Input: part model. Units: mm. Frame: model coordinates. A direction names the side the tool comes from. Round coordinates to 2 decimals unless told otherwise and drop trailing zeros. Loops run counter-clockwise (first coordinate to the right, second up) from the corner with the lowest first, then second, coordinate; pieces in that order, holes last. Notation, with made-up numbers: (43.5, 84.25) -> (56.5, 84.25) arc R27 cw to (56.5, 100.25) -> close; hole circle Ø5 at (6.25, 15.5). An arc over 180 degrees is marked (long way). Answer as a JSON object with one key per item and string values.
```python
from build123d import *

# Parameters (mm, degrees)
SKETCH_1_R               = 100
SKETCH_1_R_2             = 80
EXTRUDE_1_DEPTH          = 10
SKETCH_3_R               = 1.6
CUT_EXTRUDE_2_DEPTH      = 142.774468788
CUT_EXTRUDE_3_DEPTH      = 3
PATTERN_CIRCULAR_1_COUNT = 3


with BuildPart() as part:
    # 草图1 → 凸台-拉伸1 (new body)
    with BuildSketch(Plane(origin=(0, 0, 0), x_dir=(1, 0, 0), z_dir=(0, 1, 0))):
        with Locations(Location((0, 0, 0), (0, 0, 270))):
            Circle(SKETCH_1_R)
        with Locations(Location((0, 0, 0), (0, 0, 270))):
            Circle(SKETCH_1_R_2, mode=Mode.SUBTRACT)
    extrude(amount=EXTRUDE_1_DEPTH)

    # 草图3 → 切除-拉伸2 (cut, through all)
    with BuildSketch(Plane(origin=(0, 10, 0), x_dir=(1, 0, 0), z_dir=(0, 1, 0))):
        with Locations(Location((-62.39260708, 68.252564653, 0), (0, 0, 270))):
            Circle(SKETCH_3_R)
        with Locations(Location((-84.573353466, 37.397832605, 0), (0, 0, 270))):
            Circle(SKETCH_3_R)
    cut_extrude_2 = extrude(amount=-CUT_EXTRUDE_2_DEPTH, mode=Mode.SUBTRACT)

    # 草图4 → 切除-拉伸3 (cut)
    with BuildSketch(Plane.XZ):
        Polygon((-80.877120495, -38.81834724), (-83.152838831, -33.701599634), (-88.269586436, -35.97731797), (-85.993868101, -41.094065575), align=None)
        Polygon((-62.126188983, -72.20339006), (-66.343432487, -68.51898275), (-62.659025177, -64.301739246), (-58.441781673, -67.986146556), align=None)
    cut_extrude_3 = extrude(amount=-CUT_EXTRUDE_3_DEPTH, mode=Mode.SUBTRACT)

    # 阵列(圆周)1: 切除-拉伸2, 切除-拉伸3 ×3 about axis
    pattern_circular_1_axis = Axis((0, 0, 0), (0, 1, 0))
    add([cut_extrude_2.rotate(pattern_circular_1_axis, i * 360 / PATTERN_CIRCULAR_1_COUNT) for i in range(1, PATTERN_CIRCULAR_1_COUNT)], mode=Mode.SUBTRACT)
    add([cut_extrude_3.rotate(pattern_circular_1_axis, i * 360 / PATTERN_CIRCULAR_1_COUNT) for i in range(1, PATTERN_CIRCULAR_1_COUNT)], mode=Mode.SUBTRACT)


solid = part.part
```
1) Contact query for flat-ended pins moving along their axis: P1, Ø2, axis at x = -28, z = 90, coming from the -Y side; P2, Ø4, axis at y = 7.5, z = 38.5, coming from the -X side; P3, Ø2, axis at x = -57.5, z = 76, coming from the -Y side; P4, Ø4, axis at x = 54, y = 4.5, coming from the -Z side. Output: stop coordinate, or through.
Output:
{"P1": "stops at y = 3", "P2": "stops at x = -93.1", "P3": "stops at y = 0", "P4": "stops at z = -85.42"}
2) Section B-B, the plane x = 0. Output: boundary loops of the cut face in (y, z), plus the area to 3 significant figures.
Output:
{"outline": "(0, -100) -> (10, -100) -> (10, -80) -> (0, -80) -> close; (0, 80) -> (10, 80) -> (10, 100) -> (0, 100) -> close", "area": "400 mm^2"}
3) Reachability of faces 1 (the face through (-78.1, 4.93, -17.34)), 2 (the face through (-27, 3, 90)) from +Z, -Z, +X, -X, +Y, -Y: full face, straight path, thin tool, end or side. Return the list, or none.
Output:
{"face 1": "+Y, -Y", "face 2": "-Y"}
4) Section C-C, the plane y = 5.25. Output: boundary loops of the cut face in (x, z).
Output:
{"outline": "circle Ø200 at (0, 0); hole circle Ø3.2 at (-84.57, -37.4); hole circle Ø160 at (0, 0); hole circle Ø3.2 at (-62.39, -68.25); hole circle Ø3.2 at (-27.91, 88.16); hole circle Ø3.2 at (9.9, 91.94); hole circle Ø3.2 at (74.67, -54.54); hole circle Ø3.2 at (90.3, -19.91)"}
5) Section A-A, the plane z = 0. Output: boundary loops of the cut face in (x, y), plus the area to 3 significant figures.
Output:
{"outline": "(-100, 0) -> (-80, 0) -> (-80, 10) -> (-100, 10) -> close; (80, 0) -> (100, 0) -> (100, 10) -> (80, 10) -> close", "area": "400 mm^2"}
6) Ray query, probe 1 along Z at (x, y) = (2, 5.75) (3 decimals); probe 2 along X at (y, z) = (0.5, 89.5); probe 3 along X at (y, z) = (1.25, -41). Return the intervals inside material, ascending.
Output:
{"probe 1": "z = -99.98 to -79.975, 79.975 to 99.98", "probe 2": "x = -44.61 to -31.33, -25.41 to 6.83, 12.46 to 44.61", "probe 3": "x = -91.21 to -86.04, -85.78 to -68.69, 68.69 to 91.21"}
7) Draft query along X for faces 3 (the face through (73, 3, -54)), 4 (the face through (45, 10, -67)), 5 (the face through (30.04, 4.93, 95.38)). Return one class per face: +X half, -X half, draft (parallel to the pull), parting line (faces both ways), or undercut.
Output:
{"face 3": "undercut", "face 4": "draft", "face 5": "parting line"}
